from build123d import *

# Parameters (mm, degrees)
SKETCH_1_W          = 30
SKETCH_1_H          = 110
SKETCH_1_R          = 1.25
EXTRUDE_1_DEPTH     = 2
FILLET_1_R          = 1
FILLET_2_R          = 18
SKETCH_2_W          = 23
SKETCH_2_H          = 50
EXTRUDE_2_DEPTH     = 2
SKETCH_3_W          = 132.5
SKETCH_3_H          = 30
EXTRUDE_3_DEPTH     = 2
FILLET_3_R          = 16
SKETCH_4_W          = 10
SKETCH_4_H          = 50
EXTRUDE_4_DEPTH     = 2
FILLET_5_R          = 6
FILLET_6_R          = 2
FILLET_7_R          = 2
CUT_EXTRUDE_1_DEPTH = 10
CUT_EXTRUDE_2_DEPTH = 10
FILLET_9_R          = 10
CUT_EXTRUDE_3_DEPTH = 10
FILLET_10_R         = 3
SKETCH_8_R          = 1.5
CUT_EXTRUDE_4_DEPTH = 10


with BuildPart() as part:
    # 草图1 → 凸台-拉伸1 (new body)
    with BuildSketch(Plane(origin=(0, 0, 0), x_dir=(1, 0, 0), z_dir=(0, 1, 0))):
        Rectangle(SKETCH_1_W, SKETCH_1_H)
        with Locations(Location((13, 27, 0), (0, 0, 270))):
            Circle(SKETCH_1_R, mode=Mode.SUBTRACT)
        with Locations(Location((-13, 27, 0), (0, 0, 90))):
            Circle(SKETCH_1_R, mode=Mode.SUBTRACT)
        with Locations(Location((-13, -27, 0), (0, 0, 270))):
            Circle(SKETCH_1_R, mode=Mode.SUBTRACT)
        with Locations(Location((13, -27, 0), (0, 0, 90))):
            Circle(SKETCH_1_R, mode=Mode.SUBTRACT)
        with Locations(Location((13, 53, 0), (0, 0, 270))):
            Circle(SKETCH_1_R, mode=Mode.SUBTRACT)
        with Locations(Location((13, -53, 0), (0, 0, 90))):
            Circle(SKETCH_1_R, mode=Mode.SUBTRACT)
    extrude(amount=EXTRUDE_1_DEPTH)

    # 圆角1
    fillet_1_edges = [part.edges().sort_by_distance(p)[0] for p in [
        (15, 1, 55),
        (15, 1, -55),
    ]]
    fillet(fillet_1_edges, radius=FILLET_1_R)

    # 圆角2
    fillet_2_edges = [part.edges().sort_by_distance(p)[0] for p in [
        (-15, 1, 55),
        (-15, 1, -55),
    ]]
    fillet(fillet_2_edges, radius=FILLET_2_R)

    # 草图2 → 凸台-拉伸2 (add)
    with BuildSketch(Plane(origin=(0, 2, 0), x_dir=(1, 0, 0), z_dir=(0, 1, 0))):
        with Locations((-26.5, -12)):
            Rectangle(SKETCH_2_W, SKETCH_2_H)
    extrude(amount=-EXTRUDE_2_DEPTH)

    # 草图3 → 凸台-拉伸3 (add)
    with BuildSketch(Plane(origin=(0, 2, 0), x_dir=(1, 0, 0), z_dir=(0, 1, 0))):
        with Locations((81.25, -7)):
            Rectangle(SKETCH_3_W, SKETCH_3_H)
    extrude(amount=-EXTRUDE_3_DEPTH)

    # 圆角3
    fillet_3_edges = [part.edges().sort_by_distance(p)[0] for p in [
        (15, 1, 22),
        (15, 1, -8),
    ]]
    fillet(fillet_3_edges, radius=FILLET_3_R)

    # 草图4 → 凸台-拉伸4 (add)
    with BuildSketch(Plane.XZ):
        with Locations((142.5, 12)):
            Rectangle(SKETCH_4_W, SKETCH_4_H)
    extrude(amount=-EXTRUDE_4_DEPTH)

    # 圆角5
    fillet_5_edges = [part.edges().sort_by_distance(p)[0] for p in [
        (137.5, 1, 22),
    ]]
    fillet(fillet_5_edges, radius=FILLET_5_R)

    # 圆角6
    fillet_6_edges = [part.edges().sort_by_distance(p)[0] for p in [
        (137.5, 1, -8),
    ]]
    fillet(fillet_6_edges, radius=FILLET_6_R)

    # 圆角7
    fillet_7_edges = [part.edges().sort_by_distance(p)[0] for p in [
        (147.5, 1, 37),
        (137.5, 1, -13),
        (137.5, 1, 37),
        (147.5, 1, -13),
        (-38, 1, 37),
        (-38, 1, -13),
    ]]
    fillet(fillet_7_edges, radius=FILLET_7_R)

    # 草图5 → 切除-拉伸1 (cut)
    with BuildSketch(Plane.XZ):
        with BuildLine():
            Line((-8.171572875, 29), (11, 29))
            Line((11, 29), (11, 48.171572875))
            ThreePointArc((11, 48.171572875), (-5.055430247, 45.055430247), (-8.171572875, 29))
        make_face()
        with BuildLine():
            Line((11, -29), (11, -48.171572875))
            ThreePointArc((11, -48.171572875), (-5.055430247, -45.055430247), (-8.171572875, -29))
            Line((-8.171572875, -29), (11, -29))
        make_face()
    extrude(amount=-CUT_EXTRUDE_1_DEPTH, mode=Mode.SUBTRACT)

    # 草图6 → 切除-拉伸2 (cut)
    with BuildSketch(Plane.XZ):
        with BuildLine():
            Line((-5, -18), (-5, 18))
            ThreePointArc((-5, 18), (0, 23), (5, 18))
            Line((5, 18), (5, -18))
            ThreePointArc((5, -18), (0, -23), (-5, -18))
        make_face()
    extrude(amount=-CUT_EXTRUDE_2_DEPTH, mode=Mode.SUBTRACT)

    # 圆角9
    fillet_9_edges = [part.edges().sort_by_distance(p)[0] for p in [
        (-15, 1, 37),
        (-15, 1, -13),
    ]]
    fillet(fillet_9_edges, radius=FILLET_9_R)

    # 草图7 → 切除-拉伸3 (cut)
    with BuildSketch(Plane.XZ):
        with BuildLine():
            Line((24.271968642, 12), (124.271968642, 12))
            ThreePointArc((124.271968642, 12), (129.271968642, 7), (124.271968642, 2))
            Line((124.271968642, 2), (24.271968642, 2))
            ThreePointArc((24.271968642, 2), (19.271968642, 7), (24.271968642, 12))
        make_face()
    extrude(amount=-CUT_EXTRUDE_3_DEPTH, mode=Mode.SUBTRACT)

    # 圆角10
    fillet_10_edges = [part.edges().sort_by_distance(p)[0] for p in [
        (-8.171572875, 1, 29),
        (11, 1, 48.171572875),
        (11, 1, 29),
        (11, 1, -48.171572875),
        (-8.171572875, 1, -29),
        (11, 1, -29),
    ]]
    fillet(fillet_10_edges, radius=FILLET_10_R)

    # 草图8 → 切除-拉伸4 (cut)
    with BuildSketch(Plane.XZ):
        with Locations(Location((-35, 17, 0), (0, 0, 270))):
            Circle(SKETCH_8_R)
        with Locations(Location((-35, -3, 0), (0, 0, 270))):
            Circle(SKETCH_8_R)
        with Locations(Location((144.5, 17, 0), (0, 0, 270))):
            Circle(SKETCH_8_R)
        with Locations(Location((144.5, -3, 0), (0, 0, 270))):
            Circle(SKETCH_8_R)
    extrude(amount=-CUT_EXTRUDE_4_DEPTH, mode=Mode.SUBTRACT)


solid = part.part
Work out the finished part from the listing and answer in its coordinate system (mm). A direction names the side the tool comes from. Round coordinates to 2 decimals unless told otherwise and drop trailing zeros. Order: outer loops, then holes, each group sorted by start corner. A loop starts at its lowest first (then second) coordinate and runs counter-clockwise, first axis right, second up. Notation, with made-up numbers: M 59,12 L 111,12 A27 cw 111,39 Z; hole C -15.75,23 d7. An arc over 180 degrees is marked long. Put each result on its own line as item: value. Start each with the question number.
Q1. Flat-ended cylindrical pins translate along their axes: pin 1 (1 mm diameter, centred on y = 1, z = -29.5, fed in from -X); pin 2 (1 mm diameter, centred on x = 67, y = 1.5, fed in from -Z); pin 3 (1 mm diameter, centred on x = 65, y = 1, fed in from +Z). Find the tip coordinate at first contact, or state that the pin passes through.
Q2. Section B-B, the plane x = 47.5 is taken. Write down the section's boundary in (y, z).
Q3. Straight lines are drawn through the part: L1, parallel to X at y = 0.5, z = -27; L2, parallel to X at y = 1.3, z = -3; L3, parallel to Z at x = 61.5, y = 0.9. For each, find the intervals that lie inside material, in ascending order. Write a range as [from, to].
Q4. A tool of negligible diameter and unlimited length cuts with its end or side. For faces 4 (the flat face through (33, 2, 1)), 5 (the cylindrical face through (-9.867, 1.014, -49.587)), 6 (the cylindrical face through (19.563, 0.986, -12.811)), 7 (the cylindrical face through (0, 1, -23)), 8 (the cylindrical face through (19.563, 0.986, 26.811)), from which of +Z, -Z, +X, -X, +Y, -Y can it reach the whole face along a straight path? Write none if from no direction.
Q5. Section C-C, the plane z = -21 is taken. Write down the section's boundary in (x, y), and give its area (3 significant figures).
Q6. Section D-D, the plane y = 1.05 is taken. Give the number of separate pieces and of enclosed holes in the cut face, and give its area (3 significant figures).
Q7. Section A-A, the plane z = 7 is taken. Write down the section's boundary in (x, y), and give its area (3 significant figures).
Q8. For a pull along X with two mould halves and no side action, classify faces 1 (the cylindrical face through (0, 1, 23)), 2 (the cylindrical face through (-17.85, 0.99, -16.01)), 3 (the flat face through (33, 0, 1)) as pulls with the +X half, pulls with the -X half, needs draft (parallel to the pull), parting line crosses it, or undercut.
Findings below:
1. pin 1: stops at x = -15
1. pin 2: stops at z = -8
1. pin 3: stops at z = 22
2. outline: M 0,-8 L 2,-8 L 2,2 L 0,2 Z; M 0,12 L 2,12 L 2,22 L 0,22 Z
3. L1: x = [-15, -14.25], [-11.75, 11.75], [14.25, 15]
3. L2: x = [-38, -36.5], [-33.5, -5], [5, 143], [146, 147.5]
3. L3: z = [-8, 2], [12, 22]
4. face 4: +Z, -Z, +X, -X, +Y
4. face 5: -Z, -X, +Y, -Y
4. face 6: -Z, +Y, -Y
4. face 7: +Y, -Y
4. face 8: +Z, +Y, -Y
5. outline: M -15.2,0 L -4,0 L -4,2 L -15.2,2 Z; M 4,0 L 15.28,0 L 15.28,2 L 4,2 Z
5. area: 45.0 mm^2
6. separate pieces: 1
6. enclosed holes: 14
6. area: 6,340 mm^2
7. outline: M -38,0 L -5,0 L -5,2 L -38,2 Z; M 5,0 L 19.27,0 L 19.27,2 L 5,2 Z; M 129.27,0 L 147.5,0 L 147.5,2 L 129.27,2 Z
7. area: 131 mm^2
8. face 1: undercut
8. face 2: pulls with the -X half
8. face 3: needs draft
